The listing builds one solid part. Answer for the finished solid, in the listing's coordinates (mm). A direction names the side the tool comes from. Give positions to 0.01 mm unless a question says otherwise; leave off trailing zeros. Order: outer loops, then holes, each group sorted by start corner. A loop starts at its lowest first (then second) coordinate and runs counter-clockwise, first axis right, second up. Notation, with made-up numbers: (-3, 82) -> (30, 82) arc R13 ccw to (30, 107) -> close; hole circle Ø11 at (83.5, 60). An arc over 180 degrees is marked (long way). Answer as a JSON object with one key per item and string values. Group by question number.
```python
from build123d import *

# Parameters (mm, degrees)
SKETCH1_W           = 37.846
SKETCH1_H           = 76.2
SKETCH1_R           = 4.1656
BOSS_EXTRUDE1_DEPTH = 6.35
CUT_EXTRUDE1_DEPTH  = 79.770822193


with BuildPart() as part:
    # Sketch1 → Boss-Extrude1 (new body)
    with BuildSketch(Plane.XY.offset(6.35)):
        with Locations((0, 38.1)):
            Rectangle(SKETCH1_W, SKETCH1_H)
        with Locations(Location((0, 57.15, 0), (0, 0, 180))):
            Circle(SKETCH1_R, mode=Mode.SUBTRACT)
        with Locations(Location((0, 19.05, 0), (0, 0, 180))):
            Circle(SKETCH1_R, mode=Mode.SUBTRACT)
    extrude(amount=-BOSS_EXTRUDE1_DEPTH)

    # Sketch2 → Cut-Extrude1 (cut, through all)
    with BuildSketch(Plane.XY.offset(6.35)):
        with BuildLine():
            Line((-4.1656, 6.7056), (-4.1656, 19.05))
            ThreePointArc((-4.1656, 19.05), (0, 23.2156), (4.1656, 19.05))
            Line((4.1656, 19.05), (4.1656, 6.7056))
            ThreePointArc((4.1656, 6.7056), (0, 2.54), (-4.1656, 6.7056))
        make_face()
    extrude(amount=-CUT_EXTRUDE1_DEPTH, mode=Mode.SUBTRACT)


solid = part.part
```
(1) Which of the six approach directions +Z, -Z, +X, -X, +Y, -Y give full straight-line access (tool end or side, diameter ignored) to faces 5 (the flat face through (-4.166, 13, 3)), 6 (the flat face through (18.923, 38, 3))?
(2) For a pull along Y with two mould halves and no side action, classify faces 1 (the cylindrical face through (0.092, 23.215, 3.219)), 2 (the flat face through (4.166, 13, 3)), 3 (the flat face through (0, 76.2, 3)), 4 (the flat face through (0, 39, 6.35)) as +Y half, -Y half, draft (parallel to the pull), parting line (faces both ways), or undercut.
(3) A cutting plane is placed at C-C (y = 55). Determine the outline of the cut face in (x, z).
(4) Find the intervals of material crossed by line 1 along Y through (x, z) = (0, 2); line 2 along X through (y, z) = (57.15, 3); line 3 along Y through (x, z) = (1, 4.25), in increasing order. Write a range as [from, to].
(5) A cutting plane is placed at A-A (x = 0). Determine the outline of the cut face in (y, z), and give its area (3 significant figures).
(6) A cutting plane is placed at B-B (z = 5.5). Determine the outline of the cut face in (x, y), and give its area (3 significant figures).
(7) A flat-ended cylindrical pin translates along its axis: pin 1 Ø5 at (x, y) = (0, 57.15) entering from -Z. Find the tip coordinate at first contact, or state that the pin passes through.
Check sheet entries:
{
 "1": {"face 5": "+Z, -Z", "face 6": "+Z, -Z, +X, +Y, -Y"},
 "2": {"face 1": "undercut", "face 2": "undercut", "face 3": "+Y half", "face 4": "draft"},
 "3": {"outline": "(-18.92, 0) -> (-3.57, 0) -> (-3.57, 6.35) -> (-18.92, 6.35) -> close; (3.57, 0) -> (18.92, 0) -> (18.92, 6.35) -> (3.57, 6.35) -> close"},
 "4": {"line 1": "y = [0, 2.54], [23.22, 52.98], [61.32, 76.2]", "line 2": "x = [-18.92, -4.17], [4.17, 18.92]", "line 3": "y = [0, 2.66], [23.09, 53.11], [61.19, 76.2]"},
 "5": {"outline": "(0, 0) -> (2.54, 0) -> (2.54, 6.35) -> (0, 6.35) -> close; (23.22, 0) -> (52.98, 0) -> (52.98, 6.35) -> (23.22, 6.35) -> close; (61.32, 0) -> (76.2, 0) -> (76.2, 6.35) -> (61.32, 6.35) -> close", "area": "300 mm2"},
 "6": {"outline": "(-18.92, 0) -> (18.92, 0) -> (18.92, 76.2) -> (-18.92, 76.2) -> close; hole (-4.17, 6.71) arc R4.17 ccw to (4.17, 6.71) -> (4.17, 19.05) arc R4.17 ccw to (-4.17, 19.05) -> close; hole circle Ø8.33 at (0, 57.15)", "area": "2,670 mm2"},
 "7": {"pin 1": "passes through"}
}
